Geometry check sheet. Reference: the model listing, model coordinates, mm. A direction names the side the tool comes from. Give positions to 0.01 mm unless a question says otherwise; leave off trailing zeros. Order: outer loops, then holes, each group sorted by start corner. A loop starts at its lowest first (then second) coordinate and runs counter-clockwise, first axis right, second up.
from build123d import *

# Parameters (mm, degrees)
BOSS_EXTRUDE2_DEPTH                      = 3
BOSS_EXTRUDE2_2_DEPTH                    = 3
SKETCH2_W                                = 4
SKETCH2_H                                = 19
BOSS_EXTRUDE3_DEPTH                      = 12.75
SKETCH3_W                                = 19
SKETCH3_H                                = 15.75
BOSS_EXTRUDE4_DEPTH                      = 0.75
SKETCH4_W                                = 19
SKETCH4_H                                = 15.75
BOSS_EXTRUDE5_DEPTH                      = 0.75
SKETCH5_W                                = 19
SKETCH5_H                                = 4
BOSS_EXTRUDE6_DEPTH                      = 11
FILLET1_R                                = 5
FILLET2_R                                = 1
CBORE_START                              = 5.6
CBORE_FOR_M3_PAN_HEAD_SCREW1_OUTLINE_R   = 3.5
CBORE_FOR_M3_PAN_HEAD_SCREW1_DEPTH       = 2.4
CBORE_START_2                            = 5
CBORE_FOR_M3_PAN_HEAD_SCREW1_2_OUTLINE_R = 1.7
CBORE_FOR_M3_PAN_HEAD_SCREW1_2_DEPTH     = 0.6
CUT_EXTRUDE1_START                       = -15.15
SKETCH8_R                                = 3.5
CUT_EXTRUDE1_DEPTH                       = 15.15
CUT_EXTRUDE2_START                       = -15.15
SKETCH9_R                                = 3.5
CUT_EXTRUDE2_DEPTH                       = 15.15


# Read off the part's stored shape, not the designer's step: CBORE for M3 Pan Head Screw1
with BuildPart() as part:
    # Sketch1 → Boss-Extrude2 (new body)
    with BuildSketch(Plane(origin=(0, 5, 0), x_dir=(1, 0, 0), z_dir=(0, 1, 0))):
        Polygon((6.998679183, -26), (0.748679183, -26), (0.748679183, -38), (10.998679183, -38), (10.998679183, -19), (6.998679183, -19), align=None)
    extrude(amount=BOSS_EXTRUDE2_DEPTH)



with BuildPart() as body_2:
    # Sketch1 → Boss-Extrude2 2 (new body)
    with BuildSketch(Plane(origin=(0, 5, 0), x_dir=(1, 0, 0), z_dir=(0, 1, 0))):
        Polygon((27.498679183, -26), (33.748679183, -26), (33.748679183, -38), (23.498679183, -38), (23.498679183, -19), (27.498679183, -19), align=None)
    extrude(amount=BOSS_EXTRUDE2_2_DEPTH)


with BuildPart() as part_1:
    add(part.part)

    add(body_2.part)  # Boss-Extrude3 merges body 2
    # Sketch2 → Boss-Extrude3 (add)
    with BuildSketch(Plane(origin=(0, 8, 0), x_dir=(1, 0, 0), z_dir=(0, 1, 0))):
        with Locations((8.998679183, -28.5)):
            Rectangle(SKETCH2_W, SKETCH2_H)
        with Locations((25.498679183, -28.5)):
            Rectangle(SKETCH2_W, SKETCH2_H)
    extrude(amount=BOSS_EXTRUDE3_DEPTH)

    # Sketch3 → Boss-Extrude4 (add)
    with BuildSketch(Plane(origin=(10.998679183, 0, 0), x_dir=(0, 0, -1), z_dir=(1, 0, 0))):
        with Locations((-28.5, 12.875)):
            Rectangle(SKETCH3_W, SKETCH3_H)
    extrude(amount=BOSS_EXTRUDE4_DEPTH)

    # Sketch4 → Boss-Extrude5 (add)
    with BuildSketch(Plane.ZY.offset(-23.498679183)):
        with Locations((28.5, 12.875)):
            Rectangle(SKETCH4_W, SKETCH4_H)
    extrude(amount=BOSS_EXTRUDE5_DEPTH)

    # Sketch5 → Boss-Extrude6 (add)
    with BuildSketch(Plane(origin=(11.748679183, 0, 0), x_dir=(0, 0, -1), z_dir=(1, 0, 0))):
        with Locations((-28.5, 18.75)):
            Rectangle(SKETCH5_W, SKETCH5_H)
    extrude(amount=BOSS_EXTRUDE6_DEPTH)

    # Fillet1
    fillet1_edges = [part_1.edges().sort_by_distance(p)[0] for p in [
        (6.998679183, 20.75, 28.5),
        (27.498679183, 20.75, 28.5),
    ]]
    fillet(fillet1_edges, radius=FILLET1_R)

    # Fillet2
    fillet2_edges = [part_1.edges().sort_by_distance(p)[0] for p in [
        (22.748679183, 16.75, 28.5),
        (11.748679183, 16.75, 28.5),
    ]]
    fillet(fillet2_edges, radius=FILLET2_R)

    # CBORE for M3 Pan Head Screw1 outline → CBORE for M3 Pan Head Screw1 (cut)
    with BuildSketch(Plane(origin=(0, 0, 0), x_dir=(1, 0, 0), z_dir=(0, 1, 0)).offset(CBORE_START)):
        with Locations((29.748679183, -32)):
            Circle(CBORE_FOR_M3_PAN_HEAD_SCREW1_OUTLINE_R)
        with Locations((4.748679183, -32)):
            Circle(CBORE_FOR_M3_PAN_HEAD_SCREW1_OUTLINE_R)
    extrude(amount=CBORE_FOR_M3_PAN_HEAD_SCREW1_DEPTH, mode=Mode.SUBTRACT)

    # CBORE for M3 Pan Head Screw1 2 outline → CBORE for M3 Pan Head Screw1 2 (cut)
    with BuildSketch(Plane(origin=(0, 0, 0), x_dir=(1, 0, 0), z_dir=(0, 1, 0)).offset(CBORE_START_2)):
        with Locations((29.748679183, -32)):
            Circle(CBORE_FOR_M3_PAN_HEAD_SCREW1_2_OUTLINE_R)
        with Locations((4.748679183, -32)):
            Circle(CBORE_FOR_M3_PAN_HEAD_SCREW1_2_OUTLINE_R)
    extrude(amount=CBORE_FOR_M3_PAN_HEAD_SCREW1_2_DEPTH, mode=Mode.SUBTRACT)

    # Sketch8 → Cut-Extrude1 (cut)
    with BuildSketch(Plane(origin=(0, 20.75, 0), x_dir=(1, 0, 0), z_dir=(0, 1, 0)).offset(CUT_EXTRUDE1_START)):
        with Locations(Location((4.748679183, -32, 0), (0, 0, 270))):
            Circle(SKETCH8_R)
    extrude(amount=CUT_EXTRUDE1_DEPTH, mode=Mode.SUBTRACT)

    # Sketch9 → Cut-Extrude2 (cut)
    with BuildSketch(Plane(origin=(0, 20.75, 0), x_dir=(1, 0, 0), z_dir=(0, 1, 0)).offset(CUT_EXTRUDE2_START)):
        with Locations(Location((29.748679183, -32, 0), (0, 0, 270))):
            Circle(SKETCH9_R)
    extrude(amount=CUT_EXTRUDE2_DEPTH, mode=Mode.SUBTRACT)


solid = part_1.part
Item 1: Gauge pin test, flat ends, axial feed: pin 1 (5.5 mm diameter, centred on x = 4.75, z = 32, fed in from +Y); pin 2 (3 mm diameter, centred on x = 4.75, z = 32, fed in from +Y); pin 3 (1.5 mm diameter, centred on x = 3, y = 7, fed in from -Z); pin 4 (8.5 mm diameter, centred on y = 9.5, z = 31, fed in from -X). Record the tip position at first contact, or that the pin passes through.
Reported:
pin 1: stops at y = 5.6
pin 2: passes through
pin 3: stops at z = 26
pin 4: stops at x = 0.75
Item 2: Draft check along X on faces 5 (the flat face through (27.499, 12, 36)), 6 (the flat face through (4, 5.6, 34)), 7 (the flat face through (6.999, 12, 36)). Enter one of: released by +X, released by -X, zero draft, split by the parting line, or undercut.
Reported:
face 5: released by +X
face 6: undercut
face 7: released by -X
Item 3: Sectioned sample at B-B (z = 25.25). Enter the section's corners in (x, y), and give its area (3 significant figures).
Reported:
outline: (7, 5) - (11.75, 5) - (11.75, 15.75) arc R1 cw to (12.75, 16.75) - (21.75, 16.75) arc R1 cw to (22.75, 15.75) - (22.75, 5) - (27.5, 5) - (27.5, 15.75) arc R5 ccw to (22.5, 20.75) - (12, 20.75) arc R5 ccw to (7, 15.75) - close
area: 183 mm2
Item 4: Sectioned sample at A-A (y = 13.5). Enter the section's corners in (x, z), and give its area (3 significant figures).
Reported:
outline: (7, 19) - (11.75, 19) - (11.75, 38) - (7, 38) - (7, 34.68) arc R3.5 cw to (7, 29.32) - close; (22.75, 19) - (27.5, 19) - (27.5, 29.32) arc R3.5 cw to (27.5, 34.68) - (27.5, 38) - (22.75, 38) - close
area: 171 mm2
Item 5: Sectioned sample at C-C (y = 17.5). Enter the section's corners in (x, z).
Reported:
outline: (7.31, 19) - (27.18, 19) - (27.18, 29.62) arc R3.5 cw to (27.18, 34.38) - (27.18, 38) - (7.31, 38) - (7.31, 34.38) arc R3.5 cw to (7.31, 29.62) - close
Item 6: Sectioned sample at D-D (x = 21). Enter the section's corners in (y, z).
Reported:
outline: (16.75, 19) - (20.75, 19) - (20.75, 38) - (16.75, 38) - close
Item 7: Scan lines: L1, parallel to X at y = 5.35, z = 32; L2, parallel to X at y = 13, z = 32; L3, parallel to Y at x = 28, z = 32. Record each from-to range of solid material in increasing order.
Reported:
L1: x = 0.75 to 3.05, 6.45 to 11.75, 22.75 to 28.05, 31.45 to 33.75
L2: x = 8.25 to 11.75, 22.75 to 26.25
L3: y = 5 to 5.6
Item 8: Set-up check for faces 1 (the flat face through (33.4, 8, 31.9)), 2 (the flat face through (1, 8, 32)), 3 (the flat face through (31, 6, 26)), 4 (the flat face through (17, 16.75, 29)): record each of +Z, -Z, +X, -X, +Y, -Y from which the full face is reachable in a straight line by a thin tool's end or side.
Reported:
face 1: +Z, -Z, +X, +Y
face 2: +Z, -Z, -X, +Y
face 3: -Z, +X, +Y, -Y
face 4: +Z, -Z, -Y
